```python
from build123d import *
from build123d import SkipClean  # not in build123d's __all__

# Parameters (mm, degrees)
F0_R      = 26
F1_DEPTH  = 26
F3_R      = 23.15
F4_DEPTH  = 21
F5_R      = 8.7
F6_DEPTH  = 12.5
F8_DEPTH  = 25
F9_R      = 7
F10_DEPTH = 5
F11_R     = 2
F12_DEPTH = 25
F13_W     = 5
F13_H     = 4.1104049385
F16_DEPTH = 25
F19_R     = 2
F20_R     = 0.5


with BuildPart() as f1:
    # F0 (on Right) → F1 (new body)
    with BuildSketch(Plane.YZ):
        Circle(F0_R)
    extrude(amount=F1_DEPTH)

    # F3 (on Right) → F4 (cut)
    with BuildSketch(Plane.YZ):
        Circle(F3_R)
    extrude(amount=F4_DEPTH, mode=Mode.SUBTRACT)

    # F5 (on offset) → F6 (join)
    with BuildSketch(Plane.YZ.offset(26)):
        Circle(F5_R)
    extrude(amount=-F6_DEPTH)

    # F7 (on offset) → F8 (cut)
    with BuildSketch(Plane.YZ.offset(26)):
        Polygon((-22.9713798889, 2.8702275171), (-7.9674337148, 4.6), (-13.9713798889, 18.4586847852), align=None)
        Polygon((-9, 21.3289123023), (0, 9.2), (9, 21.3289123023), align=None)
        Polygon((13.9713798889, 18.4586847852), (7.9674337148, 4.6), (22.9713798889, 2.8702275171), align=None)
        Polygon((22.9713798889, -2.8702275171), (7.9674337148, -4.6), (13.9713798889, -18.4586847852), align=None)
        Polygon((9, -21.3289123023), (0, -9.2), (-9, -21.3289123023), align=None)
        Polygon((-13.9713798889, -18.4586847852), (-7.9674337148, -4.6), (-22.9713798889, -2.8702275171), align=None)
    extrude(amount=-F8_DEPTH, mode=Mode.SUBTRACT)

    # F9 (on offset) → F10 (cut)
    with BuildSketch(Plane.YZ.offset(26)):
        Circle(F9_R)
    extrude(amount=-F10_DEPTH, mode=Mode.SUBTRACT)

    # F11 (on offset) → F12 (cut)
    with BuildSketch(Plane.YZ.offset(26)):
        Circle(F11_R)
    extrude(amount=-F12_DEPTH, mode=Mode.SUBTRACT)

    # F13 (on Front) → F14 (revolve)
    with BuildSketch(Plane.XZ):
        with Locations((23.5, 23.0552024692)):
            Rectangle(F13_W, F13_H)
    revolve(axis=Axis((13.1547623314, 0, 0), (1, 0, 0)))

    # F15 (on Right) → F16 (join)
    with BuildSketch(Plane.YZ):
        Polygon((12.9330127019, 21.4006350946), (12.5, 21.6506350946), (12.0669872981, 21.9006350946), (3.5669872981, 7.1782032303), (4.4330127019, 6.6782032303), align=None)
        Polygon((-3.5669872981, 7.1782032303), (-12.0669872981, 21.9006350946), (-12.5, 21.6506350946), (-12.9330127019, 21.4006350946), (-4.4330127019, 6.6782032303), align=None)
        Polygon((-8, 0.5), (-25, 0.5), (-25, 0), (-25, -0.5), (-8, -0.5), align=None)
        Polygon((-4.4330127019, -6.6782032303), (-12.9330127019, -21.4006350946), (-12.5, -21.6506350946), (-12.0669872981, -21.9006350946), (-3.5669872981, -7.1782032303), align=None)
        Polygon((3.5669872981, -7.1782032303), (12.0669872981, -21.9006350946), (12.5, -21.6506350946), (12.9330127019, -21.4006350946), (4.4330127019, -6.6782032303), align=None)
        Polygon((8, -0.5), (25, -0.5), (25, 0), (25, 0.5), (8, 0.5), align=None)
    extrude(amount=F16_DEPTH)

    # F17 (on Front) → F18 (revolve, cut)
    with BuildSketch(Plane.XZ):
        Polygon((14.5, 23.15), (-3.0704529053, 23.15), (-1.8057800443, 5.6787895144), (13.5, 5.6787895144), (13.5, 8.7), (14.5, 8.7), align=None)
    with SkipClean():  # cleaning this boolean's faces spoils the solid; the shape is the same uncleaned
        revolve(axis=Axis((9.9325310439, 0, 0), (1, 0, 0)), mode=Mode.SUBTRACT)

    # F19
    f19_edges = [f1.edges().sort_by_distance(p)[0] for p in [
        (23.5, -7.967434, 4.6),
        (23.5, 0, 9.2),
        (23.5, 7.967434, 4.6),
        (23.5, 7.967434, -4.6),
        (23.5, 0, -9.2),
        (23.5, -7.967434, -4.6),
    ]]
    fillet(f19_edges, radius=F19_R)

    # F20
    f20_edges = [f1.edges().sort_by_distance(p)[0] for p in [
        (23.5, 20.766266, -3.12445),
        (23.5, 13.088986, -16.421889),
        (23.5, 20.766266, 3.12445),
        (23.5, 13.088986, 16.421889),
        (23.5, 7.67728, -19.546339),
        (23.5, 7.67728, 19.546339),
        (23.5, -7.67728, 19.546339),
        (23.5, -13.088986, 16.421889),
        (23.5, -20.766266, 3.12445),
        (23.5, -20.766266, -3.12445),
        (23.5, -13.088986, -16.421889),
        (23.5, -7.67728, -19.546339),
    ]]
    fillet(f20_edges, radius=F20_R)


solid = f1.part
```
The listing builds one solid part. Answer for the finished solid, in the listing's coordinates (mm). A direction names the side the tool comes from. Give positions to 0.01 mm unless a question says otherwise; leave off trailing zeros. Order: outer loops, then holes, each group sorted by start corner. A loop starts at its lowest first (then second) coordinate and runs counter-clockwise, first axis right, second up. Notation, with made-up numbers: M -29,29.25 L 19,29.25 A30 cw 19,65.25 Z; hole C -29.5,66.5 d2. An arc over 180 degrees is marked long. Put each result on its own line as item: value. Start each with the question number.
Item 1: Flat-ended cylindrical pins translate along their axes: P1, Ø3, axis at x = 17.5, y = 19, coming from the +Z side; P2, Ø2, axis at x = 4.5, y = 3, coming from the +Z side; P3, Ø17, axis at y = -3, z = -13, coming from the -X side; P4, Ø5.5, axis at y = 15, z = 9, coming from the -X side. Find the tip coordinate at first contact, or state that the pin passes through.
Item 2: Which of the six approach directions +Z, -Z, +X, -X, +Y, -Y give full straight-line access (tool end or side, diameter ignored) to faces 1 (the face through (23.535, 6.466, -2.681)), 2 (the face through (21, 13.92, 3.76)), 3 (the face through (23.535, -10.958, -11.504))?
Item 3: The part is cut by section A-A, the plane x = 19. Determine the outline of the cut face in (y, z), and give its area (3 significant figures).
Item 4: The part is cut by section B-B, the plane y = 0. Determine the outline of the cut face in (x, z), and give its area (3 significant figures).
Item 5: The part is cut by section C-C, the plane z = -13.5. Determine the outline of the cut face in (x, y), and give its area (3 significant figures).
Item 6: Find the intervals of material crossed by line 1 along Z through (x, y) = (24.45, 0); line 2 along Z through (x, y) = (18.75, 0); line 3 along Y through (x, z) = (15, -15.5), in increasing order.
Item 7: The part is cut by section D-D, the plane x = 9.25. Determine the outline of the cut face in (y, z).
Item 8: For a pull along Z with two mould halves and no side action, classify faces 4 (the face through (12.818, -20.633, -15.821)), 5 (the face through (26, 5.4, -5.4)), 6 (the face through (17.704, 7.575, 14.121)) as +Z half, -Z half, draft (parallel to the pull), parting line (faces both ways), or undercut.
Answer key:
1. P1: stops at z = 19.23
1. P2: stops at z = 25.92
1. P3: stops at x = 13.5
1. P4: passes through
2. face 1: +X
2. face 2: -X
2. face 3: +X, -X
3. outline: C 0,0 d52; hole M -23.14,-0.5 A23.15 ccw -12.01,-19.79 L -4.78,-7.27 A8.7 cw -8.69,-0.5 Z; hole M -23.14,0.5 L -8.69,0.5 A8.7 cw -4.78,7.27 L -12.01,19.79 A23.15 ccw Z; hole M -11.14,-20.29 A23.15 ccw 11.14,-20.29 L 3.91,-7.77 A8.7 cw -3.91,-7.77 Z; hole M -11.14,20.29 L -3.91,7.77 A8.7 cw 3.91,7.77 L 11.14,20.29 A23.15 ccw Z; hole C 0,0 d4; hole M 4.78,-7.27 L 12.01,-19.79 A23.15 ccw 23.14,-0.5 L 8.69,-0.5 A8.7 cw Z; hole M 4.78,7.27 A8.7 cw 8.69,0.5 L 23.14,0.5 A23.15 ccw 12.01,19.79 Z
3. area: 752 mm²
4. outline: M 0,-26 L 26,-26 L 26,-21 L 21,-21 L 21,-23.15 L 0,-23.15 Z; M 0,23.15 L 21,23.15 L 21,21 L 26,21 L 26,26 L 0,26 Z; M 13.5,-8.7 L 21,-8.7 L 21,-10.56 L 26,-10.56 L 26,-7 L 21,-7 L 21,-2 L 13.5,-2 Z; M 13.5,2 L 21,2 L 21,7 L 26,7 L 26,10.56 L 21,10.56 L 21,8.7 L 13.5,8.7 Z
4. area: 306 mm²
5. outline: M 0,-22.22 L 26,-22.22 L 26,-16.09 L 21,-16.09 L 21,-18.81 L 0,-18.81 Z; M 0,18.81 L 21,18.81 L 21,16.09 L 26,16.09 L 26,22.22 L 0,22.22 Z; M 14.5,-8.37 L 21,-8.37 L 21,-11.82 L 26,-11.82 L 26,-3.19 L 21,-3.19 L 21,-7.22 L 14.5,-7.22 Z; M 14.5,7.22 L 21,7.22 L 21,3.19 L 26,3.19 L 26,11.82 L 21,11.82 L 21,8.37 L 14.5,8.37 Z
5. area: 306 mm²
6. line 1: z = -26 to -21, -10.56 to -7, 7 to 10.56, 21 to 26
6. line 2: z = -26 to -23.15, -8.7 to -2, 2 to 8.7, 23.15 to 26
6. line 3: y = -20.87 to -17.2, -9.53 to -8.37, 8.37 to 9.53, 17.2 to 20.87
7. outline: C 0,0 d52; hole C 0,0 d46.3
8. face 4: parting line
8. face 5: draft
8. face 6: undercut
